The model under review builds one solid part; all positions refer to its coordinate system, in mm. Round coordinates to 2 decimals unless told otherwise and drop trailing zeros. Order: outer loops, then holes, each group sorted by start corner. A loop starts at its lowest first (then second) coordinate and runs counter-clockwise, first axis right, second up.
Autodesk Inventor part; units mm, degrees
ref_plane "YZ Plane" through (0, 0, 0) normal (1, 0, 0) x (0, 1, 0)
ref_plane "XZ Plane" through (0, 0, 0) normal (0, 1, 0) x (-1, 0, 0)
ref_plane "XY Plane" through (0, 0, 0) normal (0, 0, 1) x (1, 0, 0)
sketch "Sketch1" plane through (0, 0, 0) normal (0, 0, 1) x (1, 0, 0)
  line L0 (0, 0) -> (116, 0)
  line L1 (116, 0) -> (116, -42)
  line L2 (0, 0) -> (0, -42)
  circle A0 centre (8, -8) radius 1.675
  circle A1 centre (108, -8) radius 1.675
  circle A2 centre (8, -34) radius 1.675
  circle A3 centre (108, -34) radius 1.675
  circle A4 centre (58, -70) radius 10
  circle A5 centre (58, -70) radius 14.5
  line L3 (0, -42) -> (48.9181, -81.3035)
  line L4 (116, -42) -> (67.0819, -81.3035)
  dimension "d0" = 116
  dimension "d1" = 42
  dimension "d2" = 3.35
  dimension "d3" = 8
  dimension "d4" = 8
  dimension "d7" = 100
  dimension "d10" = 26
  dimension "d13" = 42
  dimension "d14" = 20
  dimension "d15" = 29
  dimension "d16" = 70
extrude "Plate1" add sketch "Sketch1" along normal blind 3
chamfer "Corner Chamfer1" distance 3 angle 45 4 edges at (0, -42, 1.5) (0, 0, 1.5) (116, 0, 1.5) (116, -42, 1.5)
equation "\"d2\" = rivet_diameter"
equation "\"d13\" = d1"
equation "\"d17\" = Thickness"
equation "\"BendRadius\" = Thickness"
equation "\"BendReliefWidth\" = Thickness"
equation "\"BendReliefDepth\" = 0.5 * Thickness"
equation "\"CornerReliefSize\" = 4 * Thickness"
equation "\"MinimumRemnant\" = 2 * Thickness"
equation "\"TransitionRadius\" = BendRadius"
equation "\"JacobiRadiusSize\" = BendRadius"
equation "\"GapSize\" = Thickness"
equation "\"A_width\" = 46"
equation "\"A_joint_diameter\" = 16"
equation "\"A_joint_tolerance\" = 3"
equation "\"l___________\" = 0"
equation "\"l__________\" = 0"
equation "\"l_________\" = 0"
equation "\"rivet_diameter\" = 3.35"
equation "\"plate_thickness\" = 3"
equation "\"l________\" = 0"
equation "\"A_B_spacing\" = 2"
equation "\"L_Piston_Bottom\" = 21"
equation "\"L_Piston_Top\" = 25"
equation "\"thin_plate\" = 1.5"
properties part number "A_B_hinge" material "Stainless Steel"
(1) To check wall thickness, follow probe 1 along Y at (x, z) = (108, 1.95) (3 decimals); probe 2 along Y at (x, z) = (53, 1.25); probe 3 along X at (y, z) = (-77.5, 1.7). State the ranges of each line that lie inside material, in increasing order.
Data:
probe 1: y = -48.428 to -35.675, -32.325 to -9.675, -6.325 to 0
probe 2: y = -83.61 to -78.66, -61.34 to 0
probe 3: x = 44.18 to 51.39, 64.61 to 71.82
(2) Consider section B-B (y = -34). Write out the cut boundary in (x, z) (3 decimals), and give its area (3 significant figures).
Data:
outline: (0, 0) - (6.325, 0) - (6.325, 3) - (0, 3) - close; (9.675, 0) - (106.325, 0) - (106.325, 3) - (9.675, 3) - close; (109.675, 0) - (116, 0) - (116, 3) - (109.675, 3) - close
area: 328 mm2
(3) Consider section D-D (z = 0.8). State how many separate pieces and enclosed holes the cut face has, and give its area (3 significant figures).
Data:
separate pieces: 1
enclosed holes: 5
area: 7,180 mm2
(4) Consider section A-A (x = 58). Write out the cut boundary in (y, z), and give its area (4 significant figures).
Data:
outline: (-84.5, 0) - (-80, 0) - (-80, 3) - (-84.5, 3) - close; (-60, 0) - (0, 0) - (0, 3) - (-60, 3) - close
area: 193.5 mm2
(5) Consider section C-C (y = -71.5). Write out the cut boundary in (x, z).
Data:
outline: (36.72, 0) - (48.11, 0) - (48.11, 3) - (36.72, 3) - close; (67.89, 0) - (79.28, 0) - (79.28, 3) - (67.89, 3) - close
(6) Draft analysis for pull direction X (two halves, no side actions). For faces 1 (the cylindrical face through (107.78, -9.66, 1.48)), 2 (the flat face through (1, -2, 1)), 3 (the flat face through (90.698, -62.329, 1.479)), state which applies: pulls with the +X half, pulls with the -X half, needs draft (parallel to the pull), parting line crosses it, or undercut.
Data:
face 1: undercut
face 2: pulls with the -X half
face 3: pulls with the +X half
